Here's how the part is built. I have some questions about the finished solid (model axes, mm). A direction names the side the tool comes from. Coordinates: 2 decimals unless noted, no trailing zeros. Write each loop counter-clockwise with the first axis right and the second up, starting at its lowest first coordinate (ties: lowest second). Pieces come first, ordered by that corner, then holes.
(1) Imagine slicing it at C-C, the plane z = 32.5. List the corners of the cut face in (x, y) for me, plus the area to 3 significant figures.
(2) Thinking about a two-plate mould opening in Y: for faces 1 (the flat face through (20, 19.1, 31)), 2 (the flat face through (20, -19.1, 31)), 3 (the flat face through (-24, 0, 20.423)), 4 (the cylindrical face through (1.28, 29.07, 24.69)), which applies, released by +Y, released by -Y, zero draft, split by the parting line, or undercut?
(3) Imagine slicing it at D-D, the plane z = 29.5. List the corners of the cut face in (x, y) for me.
(4) Please list where these lines run through material, in increasing order: probe 1 along X at (y, z) = (0, 21.05); probe 2 along X at (y, z) = (21, 35).
(5) Which directions (+Z, -Z, +X, -X, +Y, -Y) give clear straight access to the entire face, cutting with the end or side of a thin tool? Please do faces 5 (the flat face through (17.1, -22, 31)), 6 (the flat face through (19, 20, 36.173)), 7 (the conical face through (-17.62, 20.39, 25.95)), 8 (the flat face through (-20, 19.1, 31)).
(6) For pin 1 Ø7.5 at (x, y) = (-25.5, 0) entering from +Z; pin 2 Ø5.5 at (x, z) = (-19.5, 31.5) entering from -Y; pin 3 Ø1.5 at (x, z) = (18.5, 31) entering from -Y; pin 4 Ø3 at (x, y) = (-2.5, -21.5) entering from -Z, each with a flat end and sliding along its axis, tell me the tip position at first contact or that it passes through.
(7) Imagine slicing it at A-A, the plane y = 0. List the corners of the cut face in (x, z) for me.
Solid Edge part; units mm, degrees
sketch "Sketch1" plane through (0, 0, 0) normal (-1, 0, 0) x (0, -1, 0)
  line L0 (23.6, 20.423) -> (29.1, 20.423)
  line L1 (29.1, 20.423) -> (29.1, 22.423)
  line L2 (29.1, 22.423) -> (29.1, 36.173)
  line L3 (29.1, 36.173) -> (24.6, 36.173)
  line L4 (24.6, 36.173) -> (24.6, 34.173)
  line L5 (24.6, 34.173) -> (26.6, 34.173)
  line L6 (26.6, 34.173) -> (27.1, 22.423)
  line L7 (23.6, 22.423) -> (27.1, 22.423)
  line L8 (23.6, 20.423) -> (23.6, 22.423)
  dimension "D1" = 29.1
  dimension "D2" = 29.1
  dimension "D3" = 23.6
  dimension "D4" = 23.6
  dimension "D5" = 24.6
  dimension "D6" = 29.1
  dimension "D7" = 24.6
  dimension "D8" = 23.6
revolve "Rotationsausprägung_1" add sketch "Sketch1" angle 360 about axis through (0, 0, 57) along (0, 0, -1)
sketch "Sketch2" plane through (0, 0, 0) normal (-1, 0, 0) x (0, -1, 0)
  line L0 (-19.1, 36.173) -> (-19.1, 25.173)
  line L1 (-19.1, 25.173) -> (19.1, 25.173)
  line L2 (19.1, 25.173) -> (19.1, 36.173)
  line L3 (19.1, 36.173) -> (-19.1, 36.173)
  dimension "D1" = 19.1
extrude "Cutout1" cut sketch "Sketch2" along normal mid plane 75
sketch "Sketch3" plane through (0, 0, 0) normal (0, -1, 0) x (1, 0, 0)
  line L0 (-17.1, 36.173) -> (-17.1, 25.173)
  line L1 (-17.1, 25.173) -> (17.1, 25.173)
  line L2 (17.1, 25.173) -> (17.1, 36.173)
  line L3 (17.1, 36.173) -> (-17.1, 36.173)
  dimension "D1" = 17.1
extrude "Extrusionsausschnitt_2" cut sketch "Sketch3" along normal mid plane 75
fillet "Verrundung_0_75_mm" radius 0.75 4 edges at (-19.6534, -21.4606, 36.173) (19.6534, -21.4606, 36.173) (19.6534, 21.4606, 36.173) (-19.6534, 21.4606, 36.173)
fillet "Verrundung_0_5_mm" radius 0.5 12 edges at (-17.8182, 19.7503, 34.173) (-20.5071, 19.1, 25.173) (-17.1, 22.2092, 25.173) (-17.1, -22.2092, 25.173) (-20.5071, -19.1, 25.173) (-17.8182, -19.7503, 34.173) (20.5071, -19.1, 25.173) (17.1, -22.2092, 25.173) (17.8182, -19.7503, 34.173) (17.8182, 19.7503, 34.173) (17.1, 22.2092, 25.173) (20.5071, 19.1, 25.173)
Recorded:
1. outline: (-21.95, -19.1) arc R29.1 ccw to (-17.1, -23.55) - (-17.1, -20.47) arc R26.67 cw to (-18.62, -19.1) - close; (-21.95, 19.1) - (-18.62, 19.1) arc R26.67 cw to (-17.1, 20.47) - (-17.1, 23.55) arc R29.1 ccw to start; (17.1, -23.55) arc R29.1 ccw to (21.95, -19.1) - (18.62, -19.1) arc R26.67 cw to (17.1, -20.47) - close; (17.1, 20.47) arc R26.67 cw to (18.62, 19.1) - (21.95, 19.1) arc R29.1 ccw to (17.1, 23.55) - close
1. area: 42.2 mm2
2. face 1: undercut
2. face 2: undercut
2. face 3: zero draft
2. face 4: split by the parting line
3. outline: (-21.95, -19.1) arc R29.1 ccw to (-17.1, -23.55) - (-17.1, -20.63) arc R26.8 cw to (-18.8, -19.1) - close; (-21.95, 19.1) - (-18.8, 19.1) arc R26.8 cw to (-17.1, 20.63) - (-17.1, 23.55) arc R29.1 ccw to start; (17.1, -23.55) arc R29.1 ccw to (21.95, -19.1) - (18.8, -19.1) arc R26.8 cw to (17.1, -20.63) - close; (17.1, 20.63) arc R26.8 cw to (18.8, 19.1) - (21.95, 19.1) arc R29.1 ccw to (17.1, 23.55) - close
4. probe 1: x = -29.1 to -23.6, 23.6 to 29.1
4. probe 2: x = -20.14 to -17.1, 17.1 to 20.14
5. face 5: +Z, +Y, -Y
5. face 6: +Z, +X, -X, +Y, -Y
5. face 7: none
5. face 8: +Z, +X, -X
6. pin 1: stops at z = 25.17
6. pin 2: stops at y = -23.55
6. pin 3: stops at y = -23.06
6. pin 4: passes through
7. outline: (-29.1, 20.42) - (-23.6, 20.42) - (-23.6, 22.42) - (-27.1, 22.42) - (-26.98, 25.17) - (-29.1, 25.17) - close; (23.6, 20.42) - (29.1, 20.42) - (29.1, 25.17) - (26.98, 25.17) - (27.1, 22.42) - (23.6, 22.42) - close
